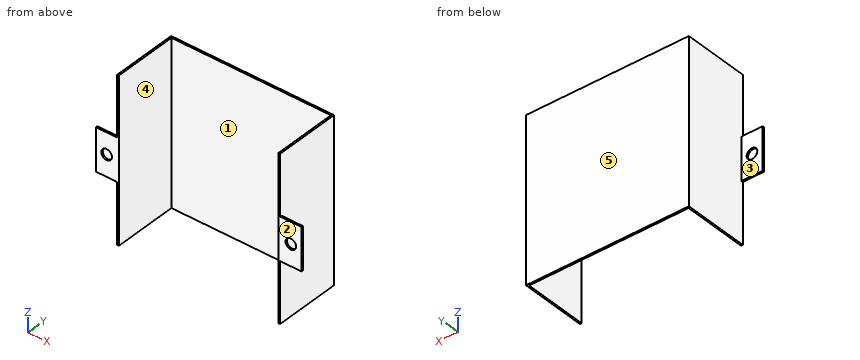
from build123d import *

# Parameters (mm, degrees)
SKETCH_1_W          = 75
SKETCH_1_H          = 75
EXTRUDE_1_DEPTH     = 0.8
SKETCH_2_W          = 76.6
SKETCH_2_H          = 76.6
SKETCH_2_W_2        = 75
SKETCH_2_H_2        = 75
EXTRUDE_2_DEPTH     = 30.8
EXTRUDE_3_DEPTH     = 0.8
F_5_0MM_1_D         = 5
SKETCH_8_W          = 75
SKETCH_8_H          = 30
CUT_EXTRUDE_1_DEPTH = 119.86631146


with BuildPart() as part:
    # 草图1 → 凸台-拉伸1 (new body)
    with BuildSketch(Plane(origin=(0, 0, 0), x_dir=(1, 0, 0), z_dir=(0, 1, 0))):
        with Locations((37.5, -37.5)):
            Rectangle(SKETCH_1_W, SKETCH_1_H)
    extrude(amount=EXTRUDE_1_DEPTH)

    # 草图2 → 凸台-拉伸2 (add)
    with BuildSketch(Plane(origin=(0, 0.8, 0), x_dir=(1, 0, 0), z_dir=(0, 1, 0))):
        with Locations((37.5, -37.5)):
            Rectangle(SKETCH_2_W, SKETCH_2_H)
        with Locations((37.5, -37.5)):
            Rectangle(SKETCH_2_W_2, SKETCH_2_H_2, mode=Mode.SUBTRACT)
    extrude(amount=-EXTRUDE_2_DEPTH)

    # 草图3 → 凸台-拉伸3 (add)
    with BuildSketch(Plane.XZ.offset(30)):
        Polygon((-0.8, 37.5), (-0.8, 47.5), (-10.8, 47.5), (-10.8, 27.5), (-0.8, 27.5), align=None)
        Polygon((75.8, 27.5), (75.8, 37.5), (75.8, 47.5), (85.8, 47.5), (85.8, 27.5), align=None)
    extrude(amount=-EXTRUDE_3_DEPTH)

    # Ø5.0mm 暗销孔1 (through all)
    with Locations(Plane(origin=(0, -30, 0), x_dir=(-1, 0, 0), z_dir=(0, -1, 0))):
        with Locations((5.8, -37.5), (-80.8, -37.5)):
            Hole(F_5_0MM_1_D / 2)

    # 草图8 → 切除-拉伸1 (cut, through all)
    with BuildSketch(Plane(origin=(0, 0, -0.8), x_dir=(-1, 0, 0), z_dir=(0, 0, -1))):
        with Locations((-37.5, -15)):
            Rectangle(SKETCH_8_W, SKETCH_8_H)
    extrude(amount=-CUT_EXTRUDE_1_DEPTH, mode=Mode.SUBTRACT)


solid = part.part
Verification items for the finished model (mm, model axes). Face numbers are marked on the shaded views. A direction names the side the tool comes from. Coordinates: 2 decimals unless noted, no trailing zeros. Write each loop counter-clockwise with the first axis right and the second up, starting at its lowest first coordinate (ties: lowest second). Pieces come first, ordered by that corner, then holes. Notation, with made-up numbers: (-39.5, 22) - (-17.5, 22) arc R14 cw to (-17.5, 44) - close; hole circle Ø7 at (35, -17). An arc over 180 degrees is marked (long way). Answer as a JSON object with one key per item and string values.
(1) Cross-section at A-A on y = -13. Record the cut outline in (x, z).
Report:
{"outline": "(-0.8, -0.8) - (0, -0.8) - (0, 75.8) - (-0.8, 75.8) - close; (75, -0.8) - (75.8, -0.8) - (75.8, 75.8) - (75, 75.8) - close"}
(2) Cross-section at D-D on z = 10.5. Record the cut outline in (x, y), plus the area to 3 significant figures.
Report:
{"outline": "(-0.8, -30) - (0, -30) - (0, 0) - (75, 0) - (75, -30) - (75.8, -30) - (75.8, 0.8) - (-0.8, 0.8) - close", "area": "109 mm^2"}
(3) Gauge pin test, flat ends, axial feed: pin 1 Ø3 at (x, z) = (79.5, 40) entering from +Y; pin 2 Ø4 at (x, z) = (10.5, 68) entering from -Y; pin 3 Ø0.9 at (x, y) = (81, -29.5) entering from -Z; pin 4 Ø4.5 at (x, z) = (-5.8, 37.5) entering from -Y. Record the tip position at first contact, or that the pin passes through.
Report:
{"pin 1": "y = -29.2", "pin 2": "y = 0", "pin 3": "z = 27.5", "pin 4": "through"}
(4) Cross-section at B-B on z = 37.5. Record the cut outline in (x, y).
Report:
{"outline": "(-10.8, -30) - (-8.3, -30) - (-8.3, -29.2) - (-10.8, -29.2) - close; (-3.3, -30) - (0, -30) - (0, 0) - (75, 0) - (75, -30) - (78.3, -30) - (78.3, -29.2) - (75.8, -29.2) - (75.8, 0.8) - (-0.8, 0.8) - (-0.8, -29.2) - (-3.3, -29.2) - close; (83.3, -30) - (85.8, -30) - (85.8, -29.2) - (83.3, -29.2) - close"}
(5) Cross-section at C-C on x = -5.8. Record the cut outline in (y, z), plus the area to 3 significant figures.
Report:
{"outline": "(-30, 27.5) - (-29.2, 27.5) - (-29.2, 35) - (-30, 35) - close; (-30, 40) - (-29.2, 40) - (-29.2, 47.5) - (-30, 47.5) - close", "area": "12.0 mm^2"}
(6) Thickness scan on line 1 along X through (y, z) = (-29.55, 37.5); line 2 along X through (y, z) = (-16, 28.5); line 3 along Z through (x, y) = (80.8, -29.6). Record the ranges inside material, lowest first.
Report:
{"line 1": "-10.8 to -8.3, -3.3 to 0, 75 to 78.3, 83.3 to 85.8", "line 2": "-0.8 to 0, 75 to 75.8", "line 3": "27.5 to 35, 40 to 47.5"}
(7) Mould release check, pull along X, two halves, no side actions. Record for the marked faces 4 and 5: pulls with the +X half, pulls with the -X half, needs draft (parallel to the pull), parting line crosses it, or undercut.
Report:
{"face 4": "undercut", "face 5": "needs draft"}
(8) Tool access check on the marked faces 1, 2 and 3. Record the directions out of +Z, -Z, +X, -X, +Y, -Y that give a thin tool (end or side, any length) a straight path to the whole face; none if there is none.
Report:
{"face 1": "+Z, -Z, -Y", "face 2": "+Z, -Z, +X, -X, -Y", "face 3": "+Z, -Z, -X, +Y"}
